```python
from build123d import *

# Parameters (mm, degrees)
F0_W          = 57.15
F0_H          = 57.15
F0_W_2        = 51.054
F0_H_2        = 51.054
F1_DEPTH      = 152.4
F2_R          = 3.048
F3_R          = 6.35
F5_DEPTH      = 28.576
F5_DEPTH_BACK = 28.576
F6_R          = 5.1562
F7_DEPTH      = 28.576
F7_DEPTH_BACK = 28.576


with BuildPart() as f1:
    # F0 (on Top) → F1 (new body)
    with BuildSketch(Plane.XY):
        Rectangle(F0_W, F0_H)
        Rectangle(F0_W_2, F0_H_2, mode=Mode.SUBTRACT)
    extrude(amount=F1_DEPTH)

    # F2
    f2_edges = [f1.edges().sort_by_distance(p)[0] for p in [
        (25.527, 25.527, 76.2),
        (-25.527, 25.527, 76.2),
        (-25.527, -25.527, 76.2),
        (25.527, -25.527, 76.2),
    ]]
    fillet(f2_edges, radius=F2_R)

    # F3
    f3_edges = [f1.edges().sort_by_distance(p)[0] for p in [
        (-28.575, 28.575, 76.2),
        (-28.575, -28.575, 76.2),
        (28.575, -28.575, 76.2),
        (28.575, 28.575, 76.2),
    ]]
    fillet(f3_edges, radius=F3_R)

    # F4 (on Front) → F5 (cut, two sides)
    with BuildSketch(Plane.XZ) as f5_sk:
        Polygon((-28.575, 152.4), (28.575, 147.4000228795), (28.575, 152.4), align=None)
    extrude(amount=-F5_DEPTH, mode=Mode.SUBTRACT)
    extrude(f5_sk.sketch, amount=F5_DEPTH_BACK, mode=Mode.SUBTRACT)

    # F6 (on Front) → F7 (cut, two sides)
    with BuildSketch(Plane.XZ) as f7_sk:
        with Locations((0, 114.3)):
            Circle(F6_R)
        with Locations((0, 38.1)):
            Circle(F6_R)
    extrude(amount=F7_DEPTH, mode=Mode.SUBTRACT)
    extrude(f7_sk.sketch, amount=-F7_DEPTH_BACK, mode=Mode.SUBTRACT)


solid = f1.part
```
Model file for the job. Use its own axes, mm. A direction names the side the tool comes from. Coordinates: 2 decimals unless noted, no trailing zeros. Loops run counter-clockwise (first coordinate to the right, second up) from the corner with the lowest first, then second, coordinate; pieces in that order, holes last. Notation, with made-up numbers: M -35,-35.5 L -11,-35.5 A23 cw -11,-22.5 Z; hole C 70,-35.5 d5. An arc over 180 degrees is marked long. Use CSV: the item, a comma, the result in double quotes. Start each with the question number.
1. Band-saw the part on A-A, the plane z = 38.1. List the corners of the cut face in (x, y) (3 decimals), then the cut area to 3 significant figures.
2. Band-saw the part on C-C, the plane x = -9.5. List the corners of the cut face in (y, z) (3 decimals).
3. Tool access for faces 1 (the cylindrical face through (2.379, 27.03, 109.726)), 2 (the flat face through (-25.527, 0, 75)): list every direction of +Z, -Z, +X, -X, +Y, -Y with a clear straight run to the whole face (end or side of a thin tool).
4. Band-saw the part on D-D, the plane z = 134. List the corners of the cut face in (x, y) (3 decimals).
5. Band-saw the part on B-B, the plane y = -1. List the corners of the cut face in (x, z) (3 decimals), then the cut area to 3 significant figures.
6. Probe probe 1 along X at (y, z) = (5, 60.5) (3 decimals); probe 2 along Z at (x, y) = (0, 27). List the from-to ranges inside material, lowest first. Write a range as [from, to].
7. Two-plate mould, pull along X, no slides. Class faces 3 (the cylindrical face through (-26.76, -26.67, 77.27)), 4 (the cylindrical face through (-24.61, -24.66, 77.13)), 5 (the cylindrical face through (-1.118, -27.03, 33.066)), 6 (the flat face through (-26, 4, 0)): pulls with the +X half, pulls with the -X half, needs draft (parallel to the pull), parting line crosses it, or undercut.
Entries:
1,outline,"M -28.575,-22.225 A6.35 ccw -22.225,-28.575 L -5.156,-28.575 L -5.156,-25.527 L -22.479,-25.527 A3.048 cw -25.527,-22.479 L -25.527,22.479 A3.048 cw -22.479,25.527 L -5.156,25.527 L -5.156,28.575 L -22.225,28.575 A6.35 ccw -28.575,22.225 Z; M 5.156,-28.575 L 22.225,-28.575 A6.35 ccw 28.575,-22.225 L 28.575,22.225 A6.35 ccw 22.225,28.575 L 5.156,28.575 L 5.156,25.527 L 22.479,25.527 A3.048 cw 25.527,22.479 L 25.527,-22.479 A3.048 cw 22.479,-25.527 L 5.156,-25.527 Z"
1,area,"570 mm2"
2,outline,"M -28.575,0 L -25.527,0 L -25.527,150.731 L -28.575,150.731 Z; M 25.527,0 L 28.575,0 L 28.575,150.731 L 25.527,150.731 Z"
3,face 1,"+Y, -Y"
3,face 2,"+Z, -Z"
4,outline,"M -28.575,-22.225 A6.35 ccw -22.225,-28.575 L 22.225,-28.575 A6.35 ccw 28.575,-22.225 L 28.575,22.225 A6.35 ccw 22.225,28.575 L -22.225,28.575 A6.35 ccw -28.575,22.225 Z; hole M -25.527,-22.479 A3.048 ccw -22.479,-25.527 L 22.479,-25.527 A3.048 ccw 25.527,-22.479 L 25.527,22.479 A3.048 ccw 22.479,25.527 L -22.479,25.527 A3.048 ccw -25.527,22.479 Z"
5,outline,"M -28.575,0 L -25.527,0 L -25.527,152.133 L -28.575,152.4 Z; M 25.527,0 L 28.575,0 L 28.575,147.4 L 25.527,147.667 Z"
5,area,"914 mm2"
6,probe 1,"x = [-28.575, -25.527], [25.527, 28.575]"
6,probe 2,"z = [0, 32.94], [43.26, 109.14], [119.46, 149.9]"
7,face 3,"pulls with the -X half"
7,face 4,"undercut"
7,face 5,"undercut"
7,face 6,"needs draft"
